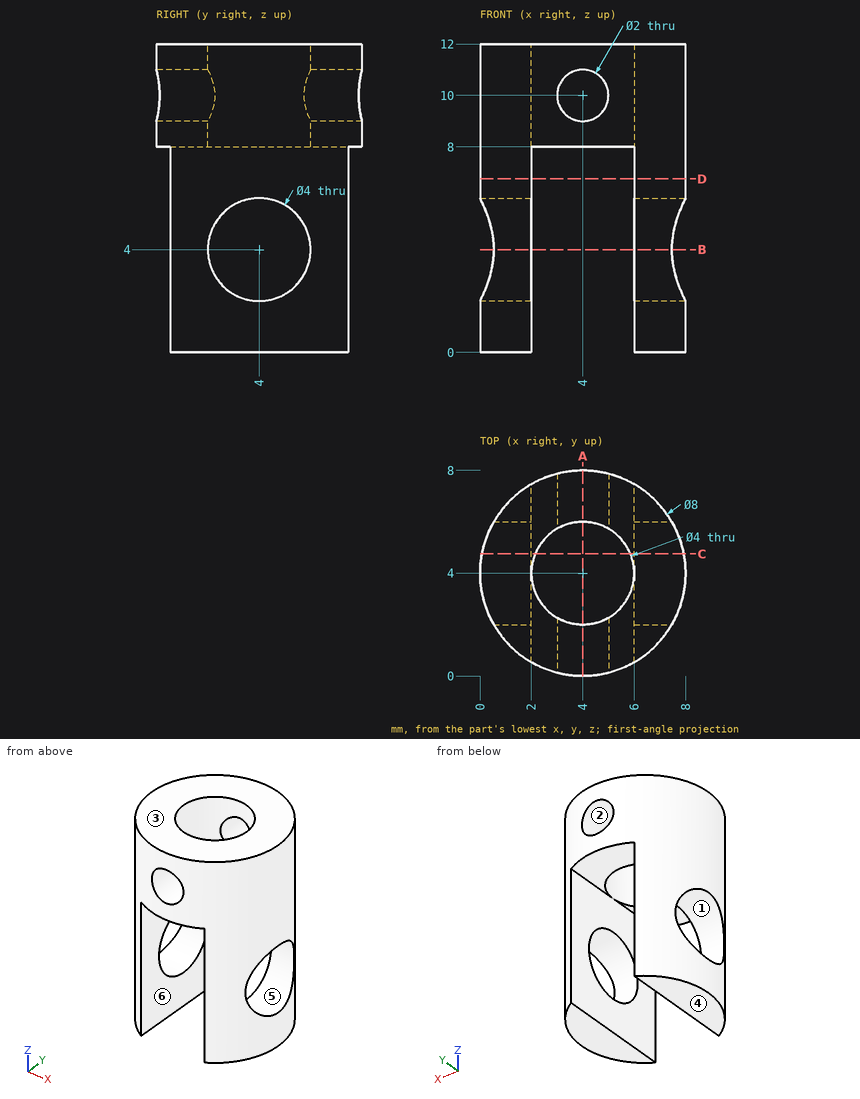
Part print with two shaded views. Sizes in mm from the minimum x, y, z corner. A direction names the side the tool comes from. Round coordinates to 2 decimals unless told otherwise and drop trailing zeros. Order: outer loops, then holes, each group sorted by start corner. A loop starts at its lowest first (then second) coordinate and runs counter-clockwise, first axis right, second up.
(1) 3-axis set-ups, long thin cutter, end or side, ignore diameter. For the marked faces 5 and 6: which of +Z, -Z, +X, -X, +Y, -Y reach the whole face in a straight line?
(2) Drill centre lines: line 1 (X direction, y = 2, z = 3.25); line 2 (Y direction, x = 4, z = 11.2); line 3 (Z direction, x = 2.5, y = 6.5). Where is each one in solid material? Low to high.
(3) Pull direction Z, two halves, no side cores. Call the marked faces 1, 2, 3 and 4: released by +Z, released by -Z, zero draft, split by the parting line, or undercut.
(4) Band-saw the part on A-A (x = 4). List the corners of the cut face in (y, z), then the cut area to 3 significant figures.
(5) Pin check, flat tip, straight feed: pin 1 (1.2 mm diameter, centred on x = 4, y = 2.5, fed in from -Z). Stop position of the tip, or through.
(6) Band-saw the part on B-B (z = 4). List the corners of the cut face in (x, y).
(7) Band-saw the part on D-D (z = 6.75). List the corners of the cut face in (x, y), then the cut area to 3 significant figures.
(8) Band-saw the part on C-C (y = 4.75). List the corners of the cut face in (x, z).
Verdict:
1. face 5: +X, -X
1. face 6: -Z, +Y, -Y
2. line 1: x = 0.54 to 2, 6 to 7.46
2. line 2: y = 0 to 2, 6 to 8
2. line 3: z = 8 to 12
3. face 1: undercut
3. face 2: undercut
3. face 3: released by +Z
3. face 4: released by -Z
4. outline: (0, 8) - (2, 8) - (2, 9) - (0, 9) - close; (0, 11) - (2, 11) - (2, 12) - (0, 12) - close; (6, 8) - (8, 8) - (8, 9) - (6, 9) - close; (6, 11) - (8, 11) - (8, 12) - (6, 12) - close
4. area: 8.00 mm2
5. pin 1: stops at z = 8
6. outline: (0.54, 2) arc R4 ccw to (2, 0.54) - (2, 2) - close; (0.54, 6) - (2, 6) - (2, 7.46) arc R4 ccw to start; (6, 0.54) arc R4 ccw to (7.46, 2) - (6, 2) - close; (6, 6) - (7.46, 6) arc R4 ccw to (6, 7.46) - close
7. outline: (2, 0.54) - (2, 7.46) arc R4 ccw to start; (6, 0.54) arc R4 ccw to (6, 7.46) - close
7. area: 19.7 mm2
8. outline: (0.07, 0) - (2, 0) - (2, 2.15) - (0.07, 2.15) - close; (0.07, 5.85) - (2, 5.85) - (2, 8) - (2.15, 8) - (2.15, 12) - (0.07, 12) - close; (5.85, 8) - (6, 8) - (6, 5.85) - (7.93, 5.85) - (7.93, 12) - (5.85, 12) - close; (6, 0) - (7.93, 0) - (7.93, 2.15) - (6, 2.15) - close
